Input: part model. Units: mm. Frame: model coordinates. Face numbers are marked on the shaded views. A direction names the side the tool comes from. Give positions to 0.01 mm unless a question says otherwise; leave off trailing zeros. Write each loop counter-clockwise with the first axis right and the second up, starting at its lowest first coordinate (ties: lowest second). Pieces come first, ordered by that corner, then holes. Notation, with made-up numbers: (-8, -18.5) - (23, -18.5) arc R9 ccw to (23, -11.5) - close; hole circle Ø10 at (2, 27.25). An arc over 180 degrees is marked (long way). Answer as a JSON object with one key per item and string values. Group by question number.
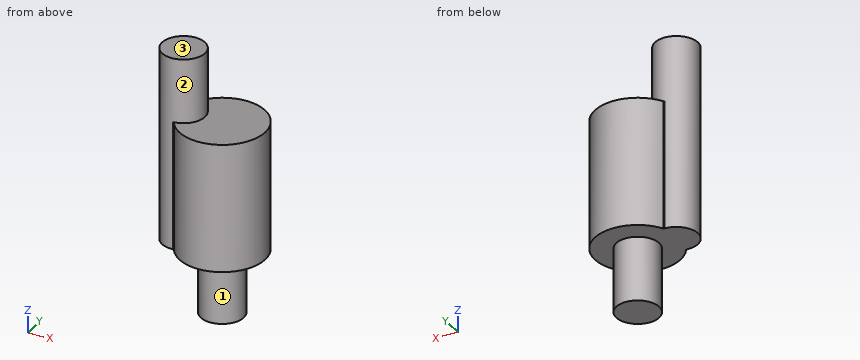
from build123d import *

# Parameters (mm, degrees)
BOSS_EXTRUDE1_DEPTH = 6
SKETCH2_R           = 1
BOSS_EXTRUDE2_DEPTH = 3
SKETCH3_R           = 1
BOSS_EXTRUDE3_DEPTH = 3


with BuildPart() as part:
    # Sketch1 → Boss-Extrude1 (new body)
    with BuildSketch(Plane.XY):
        with BuildLine():
            Line((-6.834228044, 8.847888353), (-6.766278852, 8.847888353))
            ThreePointArc((-6.766278852, 8.847888353), (-3.034228044, 7.847888353), (-6.766278852, 6.847888353))
            Line((-6.766278852, 6.847888353), (-6.834228044, 6.847888353))
            ThreePointArc((-6.834228044, 6.847888353), (-7.834228044, 7.847888353), (-6.834228044, 8.847888353))
        make_face()
    extrude(amount=BOSS_EXTRUDE1_DEPTH)

    # Sketch2 → Boss-Extrude2 (add)
    with BuildSketch(Plane.XY.offset(6)):
        with Locations(Location((-6.834228044, 7.847888353, 0), (0, 0, 270))):
            Circle(SKETCH2_R)
    extrude(amount=BOSS_EXTRUDE2_DEPTH)

    # Sketch3 → Boss-Extrude3 (add)
    with BuildSketch(Plane(origin=(0, 0, 0), x_dir=(-1, 0, 0), z_dir=(0, 0, -1))):
        with Locations(Location((5.034228044, 7.847888353, 0), (0, 0, 180))):
            Circle(SKETCH3_R)
    extrude(amount=BOSS_EXTRUDE3_DEPTH)


solid = part.part
1) Cut plane C-C on x = -5.3. Return the cut outline in (y, z).
2) Line query: line 1 along Z through (x, y) = (-4.8, 7.05); line 2 along Z through (x, y) = (-4.25, 9.2); line 3 along Y through (x, z) = (-3.4, 1.25). Output: solid intervals per line, ascending. Write a range as from..to.
3) Reachability of the marked faces 1, 2 and 3 from +Z, -Z, +X, -X, +Y, -Y: full face, straight path, thin tool, end or side. Return the list, or none.
4) Pin query (flat end, axial travel): P1, Ø1.5, axis at x = -4, z = 1.5, coming from the -Y side; P2, Ø2, axis at x = -3.5, z = 6.5, coming from the -Y side. Return the tip coordinate at first contact, or that it passes through.
5) Cut plane A-A on z = 7.5. Return the cut outline in (x, y), and give its area (3 significant figures).
6) Cut plane D-D on y = 7.6. Return the cut outline in (x, z), and give its area (3 significant figures).
7) Cut plane B-B on y = 8.35. Return the cut outline in (x, z).
Filled in:
{
 "1": {"outline": "(5.87, 0) - (6.88, 0) - (6.88, -3) - (8.81, -3) - (8.81, 0) - (9.83, 0) - (9.83, 6) - (5.87, 6) - close"},
 "2": {"line 1": "z = -3..6", "line 2": "z = 0..6", "line 3": "y = 6.69..9"},
 "3": {"face 1": "-Z", "face 2": "+Z", "face 3": "+Z, +X, -X, +Y, -Y"},
 "4": {"P1": "stops at y = 5.87", "P2": "stops at y = 5.96"},
 "5": {"outline": "circle Ø2 at (-6.83, 7.85)", "area": "3.14 mm²"},
 "6": {"outline": "(-7.8, 0) - (-6, 0) - (-6, -3) - (-4.07, -3) - (-4.07, 0) - (-3.05, 0) - (-3.05, 6) - (-5.87, 6) - (-5.87, 9) - (-7.8, 9) - close", "area": "40.1 mm²"},
 "7": {"outline": "(-7.7, 0) - (-5.9, 0) - (-5.9, -3) - (-4.17, -3) - (-4.17, 0) - (-3.1, 0) - (-3.1, 6) - (-5.97, 6) - (-5.97, 9) - (-7.7, 9) - close"}
}
